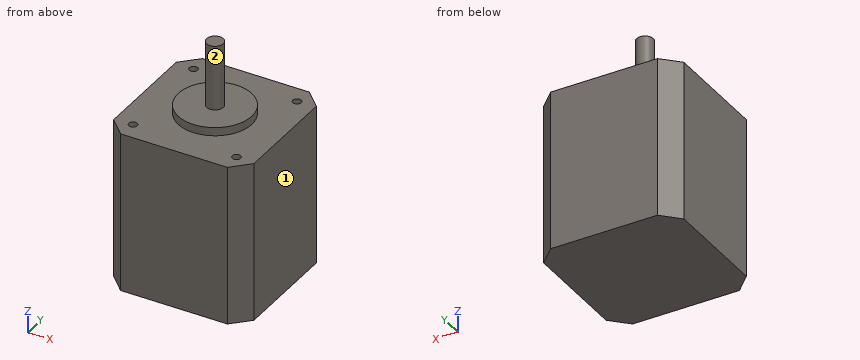
from build123d import *

# Parameters (mm, degrees)
EXTRUDE_1_DEPTH        = 24
SKETCH_2_R             = 11
SKETCH_2_R_2           = 2.5
EXTRUDE_2_DEPTH        = 2.5
SKETCH_2_2_R           = 2.5
EXTRUDE_3_DEPTH        = 22
HOLE_WIZARD_M3_1_D     = 2.5
HOLE_WIZARD_M3_1_DEPTH = 7.5
HOLE_WIZARD_M3_1_TIP   = 0.751075774


with BuildPart() as part:
    # 草图1 → 凸台-拉伸1 (new, symmetric)
    with BuildSketch(Plane.XY):
        Polygon((-21, 16), (-16, 21), (16, 21), (21, 16), (21, -16), (16, -21), (-16, -21), (-21, -16), align=None)
    extrude(amount=EXTRUDE_1_DEPTH, both=True)

    # 草图2 → 凸台-拉伸2 (add)
    with BuildSketch(Plane.XY.offset(24)):
        Circle(SKETCH_2_R)
        Circle(SKETCH_2_R_2, mode=Mode.SUBTRACT)
    extrude(amount=EXTRUDE_2_DEPTH)

    # 草图2<2> → 凸台-拉伸3 (add)
    with BuildSketch(Plane.XY.offset(24)):
        Circle(SKETCH_2_2_R)
    extrude(amount=EXTRUDE_3_DEPTH)

    # M3 螺纹孔1
    with Locations(Plane.XY.offset(24)):
        with Locations((-15.5, 15.5), (15.5, 15.5), (15.5, -15.5), (-15.5, -15.5)):
            Hole(HOLE_WIZARD_M3_1_D / 2, depth=HOLE_WIZARD_M3_1_DEPTH)
            with Locations((0, 0, -(HOLE_WIZARD_M3_1_DEPTH + HOLE_WIZARD_M3_1_TIP / 2))):  # 118° drill point
                Cone(0, HOLE_WIZARD_M3_1_D / 2, HOLE_WIZARD_M3_1_TIP, mode=Mode.SUBTRACT)


solid = part.part
The listing builds one solid part. Answer for the finished solid, in the listing's coordinates (mm). Face numbers are marked on the shaded views. A direction names the side the tool comes from. Coordinates: 2 decimals unless noted, no trailing zeros. Write each loop counter-clockwise with the first axis right and the second up, starting at its lowest first coordinate (ties: lowest second). Pieces come first, ordered by that corner, then holes. Notation, with made-up numbers: (80.25, 59) - (103.25, 59) arc R31 cw to (103.25, 94) - close; hole circle Ø2 at (87.5, 78). An arc over 180 degrees is marked (long way). Put each result on its own line as item: value.
1. The part is cut by section B-B on y = 0. Give the vertices of the cut face in (x, z).
Answer sheet:
outline: (-21, -24) - (21, -24) - (21, 24) - (11, 24) - (11, 26.5) - (2.5, 26.5) - (2.5, 46) - (-2.5, 46) - (-2.5, 26.5) - (-11, 26.5) - (-11, 24) - (-21, 24) - close
2. Flat-ended cylindrical pins translate along their axes: pin 1 Ø3 at (x, y) = (15.5, 15.5) entering from +Z; pin 2 Ø1.5 at (x, y) = (-15.5, -15.5) entering from +Z; pin 3 Ø10 at (x, y) = (10, 3.5) entering from +Z. Find the tip coordinate at first contact, or state that the pin passes through.
Answer sheet:
pin 1: stops at z = 24
pin 2: stops at z = 16.2
pin 3: stops at z = 26.5
3. A tool of negligible diameter and unlimited length cuts with its end or side. For the marked faces 1 and 2, from which of +Z, -Z, +X, -X, +Y, -Y can it reach the whole face along a straight path? Write none if from no direction.
Answer sheet:
face 1: +Z, -Z, +X, +Y, -Y
face 2: +Z
4. The part is cut by section D-D on y = -5.5. Give the vertices of the cut face in (x, z).
Answer sheet:
outline: (-21, -24) - (21, -24) - (21, 24) - (9.53, 24) - (9.53, 26.5) - (-9.53, 26.5) - (-9.53, 24) - (-21, 24) - close
5. The part is cut by section A-A on z = 13.5. Give the vertices of the cut face in (x, y).
Answer sheet:
outline: (-21, -16) - (-16, -21) - (16, -21) - (21, -16) - (21, 16) - (16, 21) - (-16, 21) - (-21, 16) - close
6. Find the intervals of material crossed by line 1 along X through (y, z) = (15.5, 20.25); line 2 along Y through (x, z) = (15, 22), in increasing order. Write a range as from..to.
Answer sheet:
line 1: x = -21..-16.75, -14.25..14.25, 16.75..21
line 2: y = -21..-16.65, -14.35..14.35, 16.65..21
